```python
from build123d import *

# Parameters (mm, degrees)
F0_R     = 12
F1_DEPTH = 5
F2_DEPTH = 75
F3_R     = 5


with BuildPart() as f1:
    # F0 (on Top) → F1 (new body)
    with BuildSketch(Plane.XY):
        with BuildLine():
            ThreePointArc((10.637082, -10.576034), (38.105118, -22), (14.477655, -3.923966))
            ThreePointArc((14.477655, -3.923966), (12.990381, 7.5), (3.840573, 14.5))
            ThreePointArc((3.840573, 14.5), (0, 44), (-3.840573, 14.5))
            ThreePointArc((-3.840573, 14.5), (-12.990381, 7.5), (-14.477655, -3.923966))
            ThreePointArc((-14.477655, -3.923966), (-38.105118, -22), (-10.637082, -10.576034))
            ThreePointArc((-10.637082, -10.576034), (0, -15), (10.637082, -10.576034))
        make_face()
        with Locations((-25.114737, -14.5)):
            Circle(F0_R, mode=Mode.SUBTRACT)
        Circle(F0_R, mode=Mode.SUBTRACT)
        with Locations((25.114737, -14.5)):
            Circle(F0_R, mode=Mode.SUBTRACT)
        with Locations((0, 29)):
            Circle(F0_R, mode=Mode.SUBTRACT)
        with Locations((25.114737, -14.5)):
            Circle(F0_R)
        Circle(F0_R)
        with Locations((0, 29)):
            Circle(F0_R)
        with Locations((-25.114737, -14.5)):
            Circle(F0_R)
    extrude(amount=F1_DEPTH)

    # F0 (on Top) → F2 (join)
    with BuildSketch(Plane.XY):
        with BuildLine():
            ThreePointArc((10.637082, -10.576034), (38.105118, -22), (14.477655, -3.923966))
            ThreePointArc((14.477655, -3.923966), (12.990381, 7.5), (3.840573, 14.5))
            ThreePointArc((3.840573, 14.5), (0, 44), (-3.840573, 14.5))
            ThreePointArc((-3.840573, 14.5), (-12.990381, 7.5), (-14.477655, -3.923966))
            ThreePointArc((-14.477655, -3.923966), (-38.105118, -22), (-10.637082, -10.576034))
            ThreePointArc((-10.637082, -10.576034), (0, -15), (10.637082, -10.576034))
        make_face()
        with Locations((-25.114737, -14.5)):
            Circle(F0_R, mode=Mode.SUBTRACT)
        Circle(F0_R, mode=Mode.SUBTRACT)
        with Locations((25.114737, -14.5)):
            Circle(F0_R, mode=Mode.SUBTRACT)
        with Locations((0, 29)):
            Circle(F0_R, mode=Mode.SUBTRACT)
    extrude(amount=F2_DEPTH)

    # F3
    f3_edges = [f1.edges().sort_by_distance(p)[0] for p in [
        (3.840573, 14.5, 37.5),
        (14.477655, -3.923966, 37.5),
        (10.637082, -10.576034, 37.5),
        (-10.637082, -10.576034, 37.5),
        (-14.477655, -3.923966, 37.5),
        (-3.840573, 14.5, 37.5),
    ]]
    fillet(f3_edges, radius=F3_R)


solid = f1.part
```
Source: CAD feature listing. Evaluate the final solid. Frame: model axes, mm. A direction names the side the tool comes from. Coordinates: 2 decimals unless noted, no trailing zeros. Loops run counter-clockwise (first coordinate to the right, second up) from the corner with the lowest first, then second, coordinate; pieces in that order, holes last. Notation, with made-up numbers: (16, -22) -> (44, -22) arc R20 cw to (44, 11) -> close; hole circle Ø1 at (39.25, 71). An arc over 180 degrees is marked (long way). One line per item, written item: value. Start each with the question number.
Q1. Section query B-B, the plane y = -23.5. Return the cut outline in (x, z), and give its area (3 significant figures).
Q2. Mould query, pull axis X, two halves, no side actions, for faces 4 (the face through (-1, 0, 0)), 5 (the face through (0.5, 43.99, 36.98)), 6 (the face through (-11.99, 29.53, 39.51)), 7 (the face through (13.02, 7.45, 36.98)). Classes: pulls with the +X half, pulls with the -X half, needs draft (parallel to the pull), parting line crosses it, or undercut.
Q3. Line query: line 1 along X through (y, z) = (-14, 56); line 2 along Y through (x, z) = (1.5, 63.5); line 3 along X through (y, z) = (29, 38). Output: solid intervals per line, ascending.
Q4. Contact query for flat-ended pins moving along their axis: P1, Ø12, axis at x = 2.5, y = 24.5, coming from the +Z side; P2, Ø19, axis at x = 0, y = 0, coming from the -Z side; P3, Ø12, axis at x = 5.5, z = 39, coming from the -Y side; P4, Ø8, axis at y = -7.5, z = 61.5, coming from the +X side. Output: stop coordinate, or through.
Q5. Set-up query: faces 1 (the face through (0, 0, 5)), 2 (the face through (0, -15, 37)), 3 (the face through (-12.96, 7.55, 36.98)). Return all of +Z, -Z, +X, -X, +Y, -Y with unobstructed straight access to the full face (end or side cutting, diameter ignored); none if empty.
Q6. Section query C-C, the plane x = -22. Return the cut outline in (y, z), and give its area (3 significant figures).
Q7. Section query D-D, the plane z = 43. Give the number of separate pieces and of enclosed holes in the cut face, and give its area (3 significant figures).
Q8. Section query A-A, the plane y = 29. Return the cut outline in (x, z), and give its area (3 significant figures).
Results:
1. outline: (-37.11, 0) -> (-13.11, 0) -> (-13.11, 75) -> (-17.18, 75) -> (-17.18, 5) -> (-33.05, 5) -> (-33.05, 75) -> (-37.11, 75) -> close; (13.11, 0) -> (37.11, 0) -> (37.11, 75) -> (33.05, 75) -> (33.05, 5) -> (17.18, 5) -> (17.18, 75) -> (13.11, 75) -> close
1. area: 1,380 mm^2
2. face 4: needs draft
2. face 5: parting line crosses it
2. face 6: undercut
2. face 7: pulls with the +X half
3. line 1: -40.11 to -37.1, -13.13 to 13.13, 37.1 to 40.11
3. line 2: -14.92 to -11.91, 11.91 to 17.09, 40.91 to 43.92
3. line 3: -15 to -12, 12 to 15
4. P1: z = 5
4. P2: z = 0
4. P3: y = -20.8
4. P4: x = 39.81
5. face 1: +Z
5. face 2: +Z, -Z, -Y
5. face 3: +Z, -Z, -X
6. outline: (-29.17, 0) -> (0.17, 0) -> (0.17, 75) -> (-2.91, 75) -> (-2.91, 5) -> (-26.09, 5) -> (-26.09, 75) -> (-29.17, 75) -> close
6. area: 579 mm^2
7. separate pieces: 1
7. enclosed holes: 4
7. area: 1,070 mm^2
8. outline: (-15, 0) -> (15, 0) -> (15, 75) -> (12, 75) -> (12, 5) -> (-12, 5) -> (-12, 75) -> (-15, 75) -> close
8. area: 570 mm^2
